Can you work these out from the model? Positions are in its coordinate system, mm. Coordinates: 2 decimals unless noted, no trailing zeros. Loops run counter-clockwise (first coordinate to the right, second up) from the corner with the lowest first, then second, coordinate; pieces in that order, holes last. Notation, with made-up numbers: M -3,-28.5 L 46,-28.5 A14 cw 46,-3.5 Z; hole C 70.25,-33.5 d8. An arc over 180 degrees is marked long. Return JSON: item names as keys, results as strings. Group by question number.
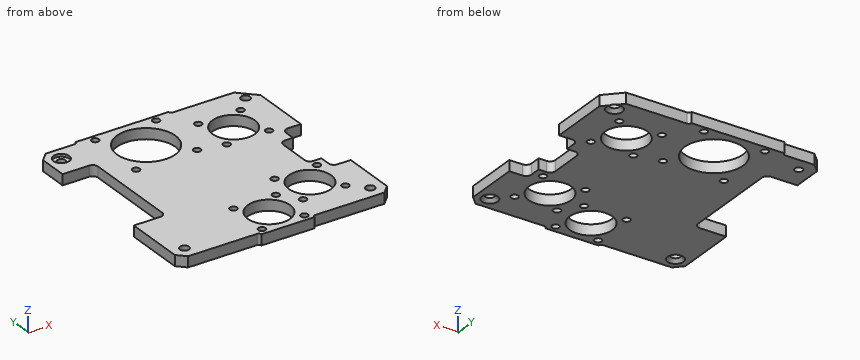
```python
from build123d import *

# Parameters (mm, degrees)
SKETCH_1_R                  = 11
SKETCH_1_R_2                = 8
EXTRUDE_1_DEPTH             = 4
SKETCH_2_R                  = 1.5
CUT_EXTRUDE_1_DEPTH         = 5
HOLE_WIZARD_2_7_2_7_1_D     = 2.7
HOLE_WIZARD_2_7_2_7_1_DEPTH = 8
HOLE_WIZARD_2_7_2_7_1_TIP   = 0.779422863
SKETCH_5_W                  = 35
SKETCH_5_H                  = 4
EXTRUDE_2_DEPTH             = 1
FILLET_1_R                  = 1
SKETCH_6_W                  = 20
SKETCH_6_H                  = 4
EXTRUDE_3_DEPTH             = 1
FILLET_2_R                  = 1
CUT_EXTRUDE_4_DEPTH         = 10
SKETCH_8_R                  = 3
CUT_EXTRUDE_5_DEPTH         = 1
HOLE_WIZARD_M31_D           = 3.4
HOLE_WIZARD_M31_CSINK_D     = 6
HOLE_WIZARD_M31_CSINK_ANGLE = 90


with BuildPart() as part:
    # Эскиз1 → Вытянуть1 (new body)
    with BuildSketch(Plane.XY):
        with BuildLine():
            Line((27.987924211, -32.908691095), (27.987924211, -9.908691095))
            Line((27.987924211, -9.908691095), (21.987924211, -3.908691095))
            Line((21.987924211, -3.908691095), (-49.012075789, -3.908691095))
            Line((-49.012075789, -3.908691095), (-52.012075789, -6.908691095))
            Line((-52.012075789, -6.908691095), (-52.012075789, -32.908691095))
            ThreePointArc((-52.012075789, -32.908691095), (-50.597862227, -33.494477533), (-50.012075789, -34.908691095))
            Line((-50.012075789, -34.908691095), (-50.012075789, -52.908691095))
            ThreePointArc((-50.012075789, -52.908691095), (-50.597862227, -54.322904658), (-52.012075789, -54.908691095))
            Line((-52.012075789, -54.908691095), (-52.012075789, -80.908691095))
            Line((-52.012075789, -80.908691095), (-49.012075789, -83.908691095))
            Line((-49.012075789, -83.908691095), (24.987924211, -83.908691095))
            Line((24.987924211, -83.908691095), (27.987924211, -80.908691095))
            Line((27.987924211, -80.908691095), (27.987924211, -54.908691095))
            ThreePointArc((27.987924211, -54.908691095), (26.573710649, -54.322904658), (25.987924211, -52.908691095))
            Line((25.987924211, -52.908691095), (25.987924211, -34.908691095))
            ThreePointArc((25.987924211, -34.908691095), (26.573710649, -33.494477533), (27.987924211, -32.908691095))
        make_face()
        with Locations((-19.785049223, -16.80111127)):
            Circle(SKETCH_1_R, mode=Mode.SUBTRACT)
        with Locations((9.413259681, -22.483355625)):
            Circle(SKETCH_1_R_2, mode=Mode.SUBTRACT)
        with Locations((-12.012075789, -74.208691095)):
            Circle(SKETCH_1_R_2, mode=Mode.SUBTRACT)
        with Locations((9.413259681, -65.334026565)):
            Circle(SKETCH_1_R_2, mode=Mode.SUBTRACT)
    extrude(amount=EXTRUDE_1_DEPTH)

    # Эскиз2 → Вырез-Вытянуть1 (cut)
    with BuildSketch(Plane.XY.offset(4)):
        with Locations((-46.660308067, -9.260458817)):
            Circle(SKETCH_2_R)
    extrude(amount=-CUT_EXTRUDE_1_DEPTH, mode=Mode.SUBTRACT)

    # Диаметр отверстия Ø2.7 (2.7)1
    with Locations(Plane(origin=(-8.285049223, -5.30111127, 4), x_dir=(1, 0, 0), z_dir=(0, 0, 1))):
        with Locations((0, 0), (0, -23), (-23, -23), (-23, 0), (25.698308904, -9.182244355), (25.698308904, -25.182244355), (9.698308904, -25.182244355), (9.698308904, -9.182244355), (25.698308904, -52.032915295), (25.698308904, -68.032915295), (9.698308904, -68.032915295), (9.698308904, -52.032915295), (4.272973434, -60.907579825), (4.272973434, -76.907579825), (-11.727026566, -60.907579825), (-11.727026566, -76.907579825)):
            Hole(HOLE_WIZARD_2_7_2_7_1_D / 2, depth=HOLE_WIZARD_2_7_2_7_1_DEPTH)
            with Locations((0, 0, -(HOLE_WIZARD_2_7_2_7_1_DEPTH + HOLE_WIZARD_2_7_2_7_1_TIP / 2))):  # 120° drill point
                Cone(0, HOLE_WIZARD_2_7_2_7_1_D / 2, HOLE_WIZARD_2_7_2_7_1_TIP, mode=Mode.SUBTRACT)

    # Эскиз5 → Вытянуть2 (add)
    with BuildSketch(Plane(origin=(0, -3.908691095, 0), x_dir=(1, 0, 0), z_dir=(0, 1, 0))):
        with Locations((-19.512075789, -2)):
            Rectangle(SKETCH_5_W, SKETCH_5_H)
    extrude(amount=EXTRUDE_2_DEPTH)

    # Скругление1
    fillet_1_edges = [part.edges().sort_by_distance(p)[0] for p in [
        (-2.012075789, -3.908691095, 2),
        (-37.012075789, -3.908691095, 2),
    ]]
    fillet(fillet_1_edges, radius=FILLET_1_R - 0.0001)  # a hair under: the kernel refuses the full size

    # Эскиз6 → Вытянуть3 (add)
    with BuildSketch(Plane.XZ.offset(83.908691095)):
        with Locations((-12.012075789, 2)):
            Rectangle(SKETCH_6_W, SKETCH_6_H)
    extrude(amount=EXTRUDE_3_DEPTH)

    # Скругление2
    fillet_2_edges = [part.edges().sort_by_distance(p)[0] for p in [
        (-2.012075789, -83.908691095, 2),
        (-22.012075789, -83.908691095, 2),
    ]]
    fillet(fillet_2_edges, radius=FILLET_2_R - 0.0001)  # a hair under: the kernel refuses the full size

    # Эскиз7 → Вытянуть4 (cut)
    with BuildSketch(Plane(origin=(0, 0, 0), x_dir=(-1, 0, 0), z_dir=(0, 0, -1))):
        with BuildLine():
            Line((52.012075789, -17.908691095), (42.012075789, -17.908691095))
            ThreePointArc((42.012075789, -17.908691095), (40.597862227, -18.494477533), (40.012075789, -19.908691095))
            Line((40.012075789, -19.908691095), (40.012075789, -55.908691095))
            ThreePointArc((40.012075789, -55.908691095), (40.597862227, -57.322904658), (42.012075789, -57.908691095))
            Line((42.012075789, -57.908691095), (52.012075789, -57.908691095))
            Line((52.012075789, -57.908691095), (52.012075789, -17.908691095))
        make_face()
        with BuildLine():
            Line((-20.987924211, -54.534916172), (-20.987924211, -58.534916172))
            ThreePointArc((-20.987924211, -58.534916172), (-21.573710649, -59.949129735), (-22.987924211, -60.534916172))
            Line((-22.987924211, -60.534916172), (-27.987924211, -60.534916172))
            Line((-27.987924211, -60.534916172), (-27.987924211, -32.534916172))
            Line((-27.987924211, -32.534916172), (-22.987924211, -32.534916172))
            ThreePointArc((-22.987924211, -32.534916172), (-21.573710649, -33.12070261), (-20.987924211, -34.534916172))
            Line((-20.987924211, -34.534916172), (-20.987924211, -38.534916172))
            Line((-20.987924211, -38.534916172), (-17.987924211, -38.534916172))
            ThreePointArc((-17.987924211, -38.534916172), (-16.573710649, -39.12070261), (-15.987924211, -40.534916172))
            Line((-15.987924211, -40.534916172), (-15.987924211, -52.534916172))
            ThreePointArc((-15.987924211, -52.534916172), (-16.573710649, -53.949129735), (-17.987924211, -54.534916172))
            Line((-17.987924211, -54.534916172), (-20.987924211, -54.534916172))
        make_face()
    extrude(amount=-CUT_EXTRUDE_4_DEPTH, mode=Mode.SUBTRACT)

    # Эскиз8 → Вытянуть5 (cut)
    with BuildSketch(Plane.XY.offset(4)):
        with Locations((-46.660308067, -9.260458817)):
            Circle(SKETCH_8_R)
    extrude(amount=-CUT_EXTRUDE_5_DEPTH, mode=Mode.SUBTRACT)

    # Зенковка для винта с потайной головкой M31 (through all)
    with Locations(Plane(origin=(22.987924211, -78.908691095, 0), x_dir=(-1, 0, 0), z_dir=(0, 0, -1))):
        with Locations((0, 0), (70, 0), (0, 70)):
            CounterSinkHole(HOLE_WIZARD_M31_D / 2, HOLE_WIZARD_M31_CSINK_D / 2, counter_sink_angle=HOLE_WIZARD_M31_CSINK_ANGLE)


solid = part.part
```
1) Suppose I cut it at B-B, the plane y = -21. List the corners of the cut face in (x, z) for me, then the cut area to 3 significant figures.
2) If I drill on line 1 (Y direction, x = -31.5, z = 3.35); line 2 (X direction, y = -58.5, z = 3.8); line 3 (X direction, y = -81, z = 1.3), over which ranges is the centre line in solid material (lowest first)? Write a range as from..to.
3) Suppose I cut it at C-C, the plane x = 15. List the corners of the cut face in (y, z) for me, then the cut area to 3 significant figures.
4) For pin 1 (2 mm diameter, centred on y = -37, z = 2.5, fed in from +X), with a flat end and sliding along its axis, tell me the tip position at first contact or that it passes through.
5) Suppose I cut it at A-A, the plane x = -28. List the corners of the cut face in (y, z) for me.
6) Suppose I cut it at D-D, the plane z = 2.3. Give the number of separate pieces and of enclosed holes in the cut face, then the cut area to 3 significant figures.
Returned:
{
 "1": {"outline": "M -40.01,0 L -29.95,0 L -29.95,4 L -40.01,4 Z; M -9.62,0 L 1.55,0 L 1.55,4 L -9.62,4 Z; M 17.27,0 L 27.99,0 L 27.99,4 L 17.27,4 Z", "area": "128 mm²"},
 "2": {"line 1": "y = -83.91..-29.63, -26.97..-6.63, -3.97..-2.91", "line 2": "x = -52.01..0.73, 2.09..5.25, 13.57..16.73, 18.09..20.99", "line 3": "x = -51.92..-20.61, -19.41..-16.24, -7.78..-4.61, -3.41..27.9"},
 "3": {"outline": "M -83.91,0 L -71.06,0 L -71.06,4 L -83.91,4 Z; M -59.61,0 L -28.21,0 L -28.21,4 L -59.61,4 Z; M -16.76,0 L -3.91,0 L -3.91,4 L -16.76,4 Z", "area": "228 mm²"},
 "4": {"pin 1": "stops at x = 20.99"},
 "5": {"outline": "M -83.91,0 L -24.12,0 L -24.12,4 L -83.91,4 Z; M -9.49,0 L -2.91,0 L -2.91,4 L -9.49,4 Z"},
 "6": {"separate pieces": "1", "enclosed holes": "24", "area": "4,560 mm²"}
}
